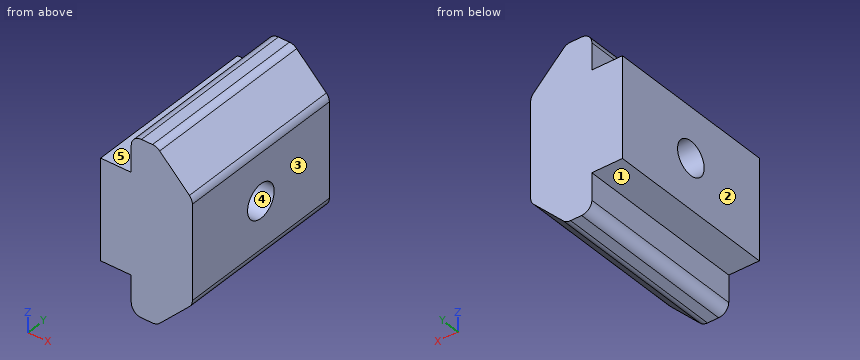
from build123d import *

# Parameters (mm, degrees)
BOSS_EXTRUDE1_DEPTH = 17
M4_TAPPED_HOLE1_D   = 3.3


with BuildPart() as part:
    # Sketch1 → Boss-Extrude1 (new body)
    with BuildSketch(Plane(origin=(0, 0, 0), x_dir=(1, 0, 0), z_dir=(0, 1, 0))):
        with BuildLine():
            Line((10.214282758, -18.266545266), (13.128495977, -15.352332485))
            ThreePointArc((13.128495977, -15.352332485), (13.345268844, -15.027908548), (13.421388977, -14.645224485))
            Line((13.421388977, -14.645224485), (13.421388977, -5.451641485))
            ThreePointArc((13.421388977, -5.451641485), (13.345268461, -5.068958498), (13.128495977, -4.744535485))
            Line((13.128495977, -4.744535485), (10.214282758, -1.830320704))
            ThreePointArc((10.214282758, -1.830320704), (9.889859409, -1.613547953), (9.507175977, -1.537427485))
            Line((9.507175977, -1.537427485), (8.421388977, -1.537427485))
            ThreePointArc((8.421388977, -1.537427485), (7.714282177, -1.830320722), (7.421388977, -2.537427537))
            Line((7.421388977, -2.537427537), (7.421388977, -5.159438485))
            Line((7.421388977, -5.159438485), (4.421388977, -5.159438485))
            Line((4.421388977, -5.159438485), (4.421388977, -14.959438485))
            Line((4.421388977, -14.959438485), (7.421388977, -14.959438485))
            Line((7.421388977, -14.959438485), (7.421388977, -17.559438537))
            ThreePointArc((7.421388977, -17.559438537), (7.714282276, -18.266545347), (8.421389151, -18.559438485))
            Line((8.421389151, -18.559438485), (9.507176151, -18.559438485))
            ThreePointArc((9.507176151, -18.559438485), (9.88985949, -18.483317984), (10.214282758, -18.266545266))
        make_face()
    extrude(amount=BOSS_EXTRUDE1_DEPTH)

    # M4 Tapped Hole1 (through all)
    with Locations(Plane.ZY.offset(-4.421388977)):
        with Locations((10.059438485, 8.5)):
            Hole(M4_TAPPED_HOLE1_D / 2)


solid = part.part
Source: CAD feature listing. Evaluate the final solid. Frame: model axes, mm. Face numbers are marked on the shaded views. A direction names the side the tool comes from. Round coordinates to 2 decimals unless told otherwise and drop trailing zeros. Loops run counter-clockwise (first coordinate to the right, second up) from the corner with the lowest first, then second, coordinate; pieces in that order, holes last.
Q1. First-contact query: P1, Ø3.5, axis at x = 6.5, y = 10.5, coming from the +Z side; P2, Ø2, axis at y = 8, z = 16, coming from the -X side; P3, Ø1.5, axis at y = 6, z = 15, coming from the -X side; P4, Ø1.5, axis at x = 5, y = 11, coming from the -Z side. Flat tips, straight axial feed; report the tip coordinate or a pass-through.
Q2. Access query for the marked faces 1 and 2. Directions: +Z, -Z, +X, -X, +Y, -Y. A direction counts if a zero-diameter tool reaches every point of the face in a straight line with its end or side. Return the directions, or none.
Q3. Section C-C, the plane y = 4.75. Return loops of the section in (x, z), plus the area to 3 significant figures.
Q4. Section D-D, the plane z = 3.75. Return loops of the section in (x, y), plus the area to 3 significant figures.
Q5. Section B-B, the plane z = 10.75. Return loops of the section in (x, y), plus the area to 3 significant figures.
Q6. Ray query, line 1 (Y direction, x = 8.25, z = 9); line 2 (Z direction, x = 6.75, y = 9); line 3 (X direction, y = 11.5, z = 14.75). Return the intervals inside material, ascending.
Q7. Section A-A, the plane y = 8.5. Return loops of the section in (x, z).
Q8. Mould query, pull axis Z, two halves, no side actions, for the marked faces 3, 4 and 5. Classes: pulls with the +Z half, pulls with the -Z half, needs draft (parallel to the pull), parting line crosses it, or undercut.
Solutions:
1. P1: stops at z = 18.54
1. P2: stops at x = 7.42
1. P3: stops at x = 4.42
1. P4: stops at z = 5.16
2. face 1: -Z, -X, +Y, -Y
2. face 2: +Z, -Z, -X, +Y, -Y
3. outline: (4.42, 5.16) - (7.42, 5.16) - (7.42, 2.54) arc R1 ccw to (8.42, 1.54) - (9.51, 1.54) arc R1 ccw to (10.21, 1.83) - (13.13, 4.74) arc R1 ccw to (13.42, 5.45) - (13.42, 14.65) arc R1 ccw to (13.13, 15.35) - (10.21, 18.27) arc R1 ccw to (9.51, 18.56) - (8.42, 18.56) arc R1 ccw to (7.42, 17.56) - (7.42, 14.96) - (4.42, 14.96) - close
3. area: 119 mm2
4. outline: (7.42, 0) - (12.13, 0) - (12.13, 17) - (7.42, 17) - close
4. area: 80.1 mm2
5. outline: (4.42, 0) - (13.42, 0) - (13.42, 7) - (4.42, 7) - close; (4.42, 10) - (13.42, 10) - (13.42, 17) - (4.42, 17) - close
5. area: 126 mm2
6. line 1: y = 0 to 7.24, 9.76 to 17
6. line 2: z = 5.16 to 8.49, 11.63 to 14.96
6. line 3: x = 4.42 to 13.42
7. outline: (4.42, 5.16) - (7.42, 5.16) - (7.42, 2.54) arc R1 ccw to (8.42, 1.54) - (9.51, 1.54) arc R1 ccw to (10.21, 1.83) - (13.13, 4.74) arc R1 ccw to (13.42, 5.45) - (13.42, 8.41) - (4.42, 8.41) - close; (4.42, 11.71) - (13.42, 11.71) - (13.42, 14.65) arc R1 ccw to (13.13, 15.35) - (10.21, 18.27) arc R1 ccw to (9.51, 18.56) - (8.42, 18.56) arc R1 ccw to (7.42, 17.56) - (7.42, 14.96) - (4.42, 14.96) - close
8. face 3: needs draft
8. face 4: undercut
8. face 5: pulls with the +Z half
